Build history of the part. All positions in model axes, mm. A direction names the side the tool comes from. Round coordinates to 2 decimals unless told otherwise and drop trailing zeros. Answer as a JSON object with one key per item and string values.
from build123d import *

# Parameters (mm, degrees)
SKETCH1_R                = 15.45
SKETCH1_R_2              = 12.45
SKETCH1_R_3              = 33
SKETCH1_R_4              = 30
SKETCH1_R_5              = 4.05
SKETCH1_R_6              = 1.05
BOSS_EXTRUDE2_DEPTH      = 12.4
BOSS_EXTRUDE3_START      = 3
SKETCH2_R                = 33
BOSS_EXTRUDE3_DEPTH      = 3
SKETCH3_R                = 33
SKETCH3_R_2              = 30
BOSS_EXTRUDE4_DEPTH      = 28.6
FILLET1_R                = 10
BOSS_EXTRUDE5_DEPTH      = 12.4
CHAMFER1_SIZE            = 4
FILLET2_R                = 5
BOSS_EXTRUDE6_DEPTH      = 28.6
BOSS_EXTRUDE6_DEPTH_BACK = 14.4
SKETCH5_R                = 4.55
SKETCH5_R_2              = 1.55
FILLET3_R                = 5
CHAMFER2_SIZE            = 2
SKETCH6_W                = 4
SKETCH6_H                = 2
CUT_EXTRUDE1_DEPTH       = 23.4


with BuildPart() as part:
    # Sketch1 → Boss-Extrude2 (new body)
    # profile 1 of 4: a face of its own
    with BuildSketch(Plane.XY):
        Circle(SKETCH1_R)
        with Locations(Location((0, 0, 0), (0, 0, 180))):
            Circle(SKETCH1_R_2, mode=Mode.SUBTRACT)
    # profile 2 of 4: a face of its own
    with BuildSketch(Plane.XY):
        with Locations(Location((0, 15.45, 0), (0, 0, 180))):
            Circle(SKETCH1_R_3)
        with Locations((0, 15.45)):
            Circle(SKETCH1_R_4, mode=Mode.SUBTRACT)
    # profile 3 of 4: a face of its own
    with BuildSketch(Plane.XY):
        with Locations(Location((11.5, 19.918584287, 0), (0, 0, 180))):
            Circle(SKETCH1_R_5)
        with Locations(Location((11.5, 19.918584287, 0), (0, 0, 180))):
            Circle(SKETCH1_R_6, mode=Mode.SUBTRACT)
    # profile 4 of 4: a face of its own
    with BuildSketch(Plane.XY):
        with Locations(Location((-11.5, 19.918584287, 0), (0, 0, 180))):
            Circle(SKETCH1_R_5)
        with Locations(Location((-11.5, 19.918584287, 0), (0, 0, 180))):
            Circle(SKETCH1_R_6, mode=Mode.SUBTRACT)
    extrude(amount=BOSS_EXTRUDE2_DEPTH)

    # Sketch2 → Boss-Extrude3 (add)
    with BuildSketch(Plane(origin=(0, 0, 0), x_dir=(-1, 0, 0), z_dir=(0, 0, -1)).offset(BOSS_EXTRUDE3_START)):
        with Locations(Location((0, 15.45, 0), (0, 0, 180))):
            Circle(SKETCH2_R)
    extrude(amount=-BOSS_EXTRUDE3_DEPTH)

    # Sketch3 → Boss-Extrude4 (add)
    with BuildSketch(Plane.XY.offset(12.4)):
        with Locations((0, 15.45)):
            Circle(SKETCH3_R)
        with Locations(Location((0, 15.45, 0), (0, 0, 256.137567884))):
            Circle(SKETCH3_R_2, mode=Mode.SUBTRACT)
    extrude(amount=BOSS_EXTRUDE4_DEPTH)

    # Fillet1
    # the kernel refuses this fillet: 10 mm, written as the material it adds along each edge
    with BuildSketch(Plane(origin=(-7.18774525, -13.676213592, 12.4), x_dir=(-0.20848530714015037, 0.9780254990063793, 0), z_dir=(0, 0, -1))) as fillet1_piece_1:
        with BuildLine():
            CenterArc((31.441766058, -6.395526036), FILLET1_R, 140.241533635, 142.62650255)
            ThreePointArc((33.668828933, -16.144381915), (14.016585538, -13.948724396), (0, 0))
            ThreePointArc((0, 0), (11.877146347, -5.568912274), (23.754292694, 0))
        make_face()
    extrude(amount=12.4)
    with BuildSketch(Plane(origin=(7.18774525, -13.676213592, 12.4), x_dir=(0.20848530714015037, 0.9780254990063793, 0), z_dir=(0, 0, -1))) as fillet1_piece_2:
        with BuildLine():
            CenterArc((31.441766058, 6.395526036), FILLET1_R, 77.131963815, 142.62650255)
            ThreePointArc((33.668828933, 16.144381915), (14.016585538, 13.948724396), (0, 0))
            ThreePointArc((0, 0), (11.877146347, 5.568912274), (23.754292694, 0))
        make_face()
    extrude(amount=12.4)

    # Sketch4 → Boss-Extrude5 (add)
    with BuildSketch(Plane.XY):
        Polygon((-15.355968184, 18.680032971), (-12.140166258, 9.556090373), (-4.457434094, 12.838952207), (4.080215127, 12.838952207), (12.140166258, 9.556090373), (15.355968184, 18.680032971), (9.70403689, 17.830268754), (8.160430255, 22.209822799), (0, 15.45), (-8.160430255, 22.209822799), (-10.090971595, 17.830268754), align=None)
    extrude(amount=BOSS_EXTRUDE5_DEPTH)

    # Chamfer1
    chamfer1_edges = [part.edges().sort_by_distance(p)[0] for p in [
        (0, 45.45, 0),
        (-23.339432443, 6.316081984, 0),
        (23.339432443, 6.316081984, 0),
    ]]
    chamfer(chamfer1_edges, length=CHAMFER1_SIZE)

    # Fillet2
    # the kernel refuses this fillet: 5 mm, written as the material it adds along each edge
    with BuildSketch(Plane(origin=(-11.5, 19.918584287, 0), x_dir=(0.4626548968458433, -0.8865384630260337, 0), z_dir=(0.8865384630260337, 0.4626548968458433, 0))) as fillet2_piece_1:
        with BuildLine():
            CenterArc((4.05 + FILLET2_R, -FILLET2_R), FILLET2_R, 90, 90)
            Line((4.05, -FILLET2_R), (4.05, 0))
            Line((4.05, 0), (4.05 + FILLET2_R, 0))
        make_face()
    revolve(axis=Axis((-11.5, 19.918584287, 0), (0, 0, -1)), revolution_arc=359.64)
    with BuildSketch(Plane(origin=(11.5, 19.918584287, 0), x_dir=(-0.4682160132284685, -0.8836140361925214, 0), z_dir=(0.8836140361925214, -0.4682160132284685, 0))) as fillet2_piece_2:
        with BuildLine():
            CenterArc((4.05 + FILLET2_R, -FILLET2_R), FILLET2_R, 90, 90)
            Line((4.05, -FILLET2_R), (4.05, 0))
            Line((4.05, 0), (4.05 + FILLET2_R, 0))
        make_face()
    revolve(axis=Axis((11.5, 19.918584287, 0), (0, 0, -1)), revolution_arc=359.64)

    # Sketch5 → Boss-Extrude6 (add, two sides: drawn at the far end of the back side and taken through both)
    # profile 1 of 3: a face of its own
    with BuildSketch(Plane.XY.offset(12.4).offset(-BOSS_EXTRUDE6_DEPTH_BACK)):
        with Locations((0, 43.45)):
            Circle(SKETCH5_R)
        with Locations((0, 43.45)):
            Circle(SKETCH5_R_2, mode=Mode.SUBTRACT)
    # profile 2 of 3: a face of its own
    with BuildSketch(Plane.XY.offset(12.4).offset(-BOSS_EXTRUDE6_DEPTH_BACK)):
        with Locations((24.248711306, 1.45)):
            Circle(SKETCH5_R)
        with Locations((24.248711306, 1.45)):
            Circle(SKETCH5_R_2, mode=Mode.SUBTRACT)
    # profile 3 of 3: a face of its own
    with BuildSketch(Plane.XY.offset(12.4).offset(-BOSS_EXTRUDE6_DEPTH_BACK)):
        with Locations((-24.248711306, 1.45)):
            Circle(SKETCH5_R)
        with Locations((-24.248711306, 1.45)):
            Circle(SKETCH5_R_2, mode=Mode.SUBTRACT)
    extrude(amount=BOSS_EXTRUDE6_DEPTH + BOSS_EXTRUDE6_DEPTH_BACK)

    # Fillet3
    fillet3_edges = [part.edges().sort_by_distance(p)[0] for p in [
        (23.612570286, -3.055310711, 26.7),
        (27.832354323, 4.25356964, 26.7),
        (-27.832354323, 4.25356964, 26.7),
        (-23.612570286, -3.055310711, 26.7),
        (4.219784038, 45.151741071, 22.5),
        (-4.219784038, 45.151741071, 22.5),
    ]]
    fillet(fillet3_edges, radius=FILLET3_R)

    # Chamfer2
    chamfer2_edges = [part.edges().sort_by_distance(p)[0] for p in [
        (-33, 15.45, -3),
    ]]
    chamfer(chamfer2_edges, length=CHAMFER2_SIZE)

    # Sketch6 → Cut-Extrude1 (cut)
    with BuildSketch(Plane.XY.offset(12.4)):
        with Locations((0, -13.034949107)):
            Rectangle(SKETCH6_W, SKETCH6_H)
    extrude(amount=-CUT_EXTRUDE1_DEPTH, mode=Mode.SUBTRACT)


solid = part.part
1) Flat gauge pins, fed straight in: pin 1 Ø1.5 at (x, z) = (6, 22.5) entering from -Y; pin 2 Ø4 at (x, z) = (3, 3.5) entering from +Y; pin 3 Ø3 at (x, y) = (-12.5, 9) entering from +Z. Where does each tip first touch, or does it go through?
Checked values:
{"pin 1": "stops at y = -17.13", "pin 2": "stops at y = 48.43", "pin 3": "stops at z = 12.4"}
2) Probe L1, parallel to Y at x = 0, z = 5; L2, parallel to Y at x = 0, z = 15; L3, parallel to Y at x = 11, z = 5. List the from-to ranges inside material, lowest first. Write a range as from..to.
Checked values:
{"L1": "y = -17.55..-14.03, 12.45..15.45, 38.9..41.9, 45..48.45", "L2": "y = -17.55..-14.55, 38.9..41.9, 45..48.45", "L3": "y = -15.66..-5.83, 5.83..19, 20.84..23.94, 43.36..46.56"}
3) Cut at A-A, the plane z = 10.5. Count the separate pieces of the cut face and the enclosed holes in it, plus the area to 3 significant figures.
Checked values:
{"separate pieces": "1", "enclosed holes": "5", "area": "1,450 mm²"}
4) Which spindle directions (+Z, -Z, +X, -X, +Y, -Y) get a long thin tool onto all of the face, cutting with end or side? Do faces 1 (the face through (0, -12.035, -1)), 2 (the face through (-13.73, 14.07, 7.76)). Say none if no direction does.
Checked values:
{"face 1": "+Z, -Z", "face 2": "+Z"}
